Design review of the part built by this model. Coordinates are the model's own, in mm. Coordinates: 2 decimals unless noted, no trailing zeros. Write each loop counter-clockwise with the first axis right and the second up, starting at its lowest first coordinate (ties: lowest second). Pieces come first, ordered by that corner, then holes. Notation, with made-up numbers: (55, 9.5) - (100, 9.5) arc R20 ccw to (100, 43.5) - close; hole circle Ø8 at (61.25, 45.25). An arc over 180 degrees is marked (long way). One line per item, written item: value.
from build123d import *

# Parameters (mm, degrees)
SKETCH1_W                    = 177.8
SKETCH1_H                    = 76.2
BOSS_EXTRUDE1_DEPTH          = 1.5875
F_1_8_0_125_DIAMETER_HOLE1_D = 3.175
F_1_4_0_25_DIAMETER_HOLE1_D  = 6.35
FILLET1_R                    = 3.175
CHAMFER1_SIZE                = 0.508


with BuildPart() as part:
    # Sketch1 → Boss-Extrude1 (new body, symmetric)
    with BuildSketch(Plane(origin=(0, 0, 0), x_dir=(1, 0, 0), z_dir=(0, 1, 0))):
        Rectangle(SKETCH1_W, SKETCH1_H)
    extrude(amount=BOSS_EXTRUDE1_DEPTH, both=True)

    # 1/8 (0.125) Diameter Hole1 (through all)
    with Locations(Plane(origin=(0, 1.5875, 0), x_dir=(1, 0, 0), z_dir=(0, 1, 0))):
        with Locations((-60.325, 31.75), (0, 31.75), (60.325, 31.75), (60.325, -31.75), (0, -31.75), (-60.325, -31.75)):
            Hole(F_1_8_0_125_DIAMETER_HOLE1_D / 2)

    # 1/4 (0.25) Diameter Hole1 (through all)
    with Locations(Plane(origin=(0, 1.5875, 0), x_dir=(1, 0, 0), z_dir=(0, 1, 0))):
        with Locations((-63.28664, -11.66114), (-53.12664, -11.66114), (-42.96664, -11.66114), (-32.80664, -11.66114), (-22.64664, -11.66114), (-12.48664, -11.66114), (18.62836, -11.66114), (28.78836, -11.66114), (38.94836, -11.66114), (49.10836, -11.66114), (59.26836, -11.66114), (69.42836, -11.66114), (-69.42836, 11.66114), (-59.26836, 11.66114), (-49.10836, 11.66114), (-38.94836, 11.66114), (-28.78836, 11.66114), (-18.62836, 11.66114), (12.48664, 11.66114), (22.64664, 11.66114), (32.80664, 11.66114), (42.96664, 11.66114), (53.12664, 11.66114), (63.28664, 11.66114)):
            Hole(F_1_4_0_25_DIAMETER_HOLE1_D / 2)

    # Fillet1
    fillet1_edges = [part.edges().sort_by_distance(p)[0] for p in [
        (-88.9, 0, 38.1),
        (88.9, 0, 38.1),
        (88.9, 0, -38.1),
        (-88.9, 0, -38.1),
    ]]
    fillet(fillet1_edges, radius=FILLET1_R)

    # Chamfer1
    chamfer1_edges = [part.edges().sort_by_distance(p)[0] for p in [
        (15.66164, 1.5875, -11.66114),
        (15.66164, -1.5875, -11.66114),
        (-15.45336, 1.5875, -11.66114),
        (-15.45336, -1.5875, -11.66114),
        (-25.61336, 1.5875, -11.66114),
        (-25.61336, -1.5875, -11.66114),
        (-35.77336, 1.5875, -11.66114),
        (-35.77336, -1.5875, -11.66114),
        (-45.93336, 1.5875, -11.66114),
        (-45.93336, -1.5875, -11.66114),
        (-56.09336, 1.5875, -11.66114),
        (-56.09336, -1.5875, -11.66114),
        (-66.25336, 1.5875, -11.66114),
        (-66.25336, -1.5875, -11.66114),
        (72.60336, 1.5875, 11.66114),
        (72.60336, -1.5875, 11.66114),
        (-58.7375, 1.5875, 31.75),
        (-58.7375, -1.5875, 31.75),
        (62.44336, 1.5875, 11.66114),
        (62.44336, -1.5875, 11.66114),
        (52.28336, 1.5875, 11.66114),
        (52.28336, -1.5875, 11.66114),
        (42.12336, 1.5875, 11.66114),
        (42.12336, -1.5875, 11.66114),
        (31.96336, 1.5875, 11.66114),
        (31.96336, -1.5875, 11.66114),
        (21.80336, 1.5875, 11.66114),
        (21.80336, -1.5875, 11.66114),
        (-9.31164, 1.5875, 11.66114),
        (-9.31164, -1.5875, 11.66114),
        (1.5875, 1.5875, 31.75),
        (1.5875, -1.5875, 31.75),
        (-19.47164, 1.5875, 11.66114),
        (-19.47164, -1.5875, 11.66114),
        (-29.63164, 1.5875, 11.66114),
        (-29.63164, -1.5875, 11.66114),
        (-39.79164, 1.5875, 11.66114),
        (-39.79164, -1.5875, 11.66114),
        (-49.95164, 1.5875, 11.66114),
        (-49.95164, -1.5875, 11.66114),
        (-60.11164, 1.5875, 11.66114),
        (-60.11164, -1.5875, 11.66114),
        (-88.9, -1.5875, 0),
        (-88.9, 1.5875, 0),
        (0, -1.5875, -38.1),
        (88.9, -1.5875, 0),
        (0, -1.5875, 38.1),
        (61.9125, 1.5875, 31.75),
        (-87.97006403, -1.5875, 37.17006403),
        (87.97006403, -1.5875, 37.17006403),
        (61.9125, -1.5875, 31.75),
        (87.97006403, -1.5875, -37.17006403),
        (-87.97006403, -1.5875, -37.17006403),
        (0, 1.5875, -38.1),
        (0, 1.5875, 38.1),
        (88.9, 1.5875, 0),
        (-87.97006403, 1.5875, 37.17006403),
        (87.97006403, 1.5875, 37.17006403),
        (87.97006403, 1.5875, -37.17006403),
        (-87.97006403, 1.5875, -37.17006403),
        (61.9125, 1.5875, -31.75),
        (61.9125, -1.5875, -31.75),
        (1.5875, 1.5875, -31.75),
        (1.5875, -1.5875, -31.75),
        (-58.7375, 1.5875, -31.75),
        (-58.7375, -1.5875, -31.75),
        (56.30164, 1.5875, -11.66114),
        (56.30164, -1.5875, -11.66114),
        (66.46164, 1.5875, -11.66114),
        (66.46164, -1.5875, -11.66114),
        (46.14164, 1.5875, -11.66114),
        (46.14164, -1.5875, -11.66114),
        (35.98164, 1.5875, -11.66114),
        (35.98164, -1.5875, -11.66114),
        (25.82164, 1.5875, -11.66114),
        (25.82164, -1.5875, -11.66114),
    ]]
    chamfer(chamfer1_edges, length=CHAMFER1_SIZE)


solid = part.part
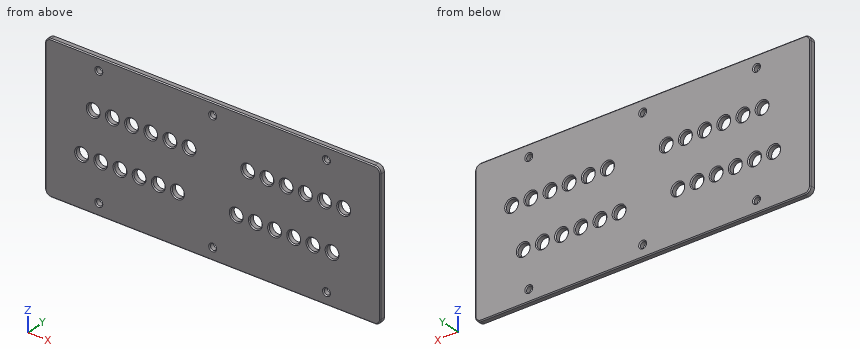
1. Consider section A-A, the plane z = 31.75. Give the number of separate pieces and of enclosed holes in the cut face, then the cut area to 3 significant figures.
Answer block:
separate pieces: 4
enclosed holes: 0
area: 532 mm^2
2. Consider section B-B, the plane x = 0. Write out the cut boundary in (y, z), then the cut area to 3 significant figures.
Answer block:
outline: (-1.59, -37.59) - (-1.08, -38.1) - (1.08, -38.1) - (1.59, -37.59) - (1.59, -33.85) - (1.08, -33.34) - (-1.08, -33.34) - (-1.59, -33.85) - close; (-1.59, -29.65) - (-1.08, -30.16) - (1.08, -30.16) - (1.59, -29.65) - (1.59, 29.65) - (1.08, 30.16) - (-1.08, 30.16) - (-1.59, 29.65) - close; (-1.59, 33.85) - (-1.08, 33.34) - (1.08, 33.34) - (1.59, 33.85) - (1.59, 37.59) - (1.08, 38.1) - (-1.08, 38.1) - (-1.59, 37.59) - close
area: 220 mm^2
3. Wall thickness on line 1 along Z through (x, y) = (23, -0.8); line 2 along Z through (x, y) = (-32.5, 0.6); line 3 along Z through (x, y) = (61, -0.4): over which ranges is each line inside the solid? List them lowest first.
Answer block:
line 1: z = -38.1 to -14.82, -8.51 to 38.1
line 2: z = -38.1 to 8.5, 14.82 to 38.1
line 3: z = -38.1 to -33.19, -30.31 to -13.86, -9.46 to 9, 14.32 to 30.31, 33.19 to 38.1
4. Insertion check: pin 1 Ø7.5 at (x, z) = (12.49, -11.66) entering from +Y. The pin has a flat end and moves straight along its axis. Give the tip position at first contact, or say it passes through.
Answer block:
pin 1: stops at y = 1.59
